Input: part model. Units: mm. Frame: model coordinates. Give positions to 0.01 mm unless a question says otherwise; leave off trailing zeros. Loops run counter-clockwise (first coordinate to the right, second up) from the corner with the lowest first, then second, coordinate; pieces in that order, holes last. Notation, with made-up numbers: (-13, 56.5) -> (4, 56.5) arc R14 cw to (4, 83.5) -> close; hole circle Ø2 at (-4, 89.25). An arc over 180 degrees is marked (long way). Answer in a Markdown table with one row per item. Add a question column.
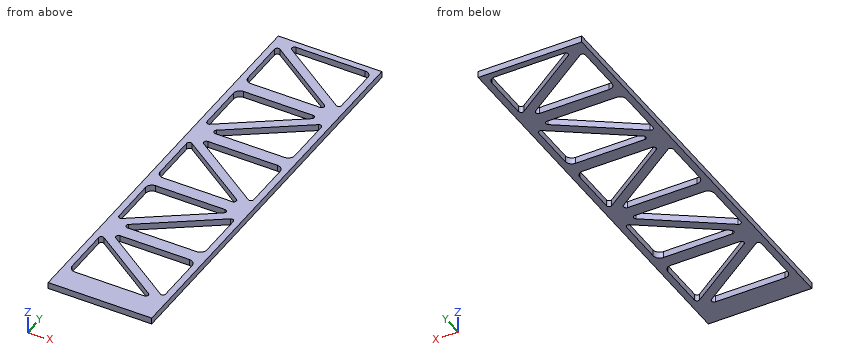
```python
from build123d import *

# Parameters (mm, degrees)
MODEL_W             = 101.6
MODEL_H             = 398.78
BOSS_EXTRUDE1_DEPTH = 6.35


with BuildPart() as part:
    # Model → Boss-Extrude1 (new body)
    with BuildSketch(Plane.XY):
        with Locations((50.8, 199.39)):
            Rectangle(MODEL_W, MODEL_H)
        with BuildLine():
            Line((88.9, 87.63), (20.83121403, 87.63))
            ThreePointArc((20.83121403, 87.63), (18.406749642, 85.847345646), (19.385420684, 83.001631833))
            Line((19.385420684, 83.001631833), (91.264206654, 33.239395393))
            ThreePointArc((91.264206654, 33.239395393), (93.888830968, 33.077884107), (95.25, 35.32776356))
            Line((95.25, 35.32776356), (95.25, 81.28))
            ThreePointArc((95.25, 81.28), (93.390128061, 85.770128061), (88.9, 87.63))
        make_face(mode=Mode.SUBTRACT)
        with BuildLine():
            Line((6.35, 157.48), (6.35, 111.52776356))
            ThreePointArc((6.35, 111.52776356), (7.711169032, 109.277884107), (10.335793346, 109.439395393))
            Line((10.335793346, 109.439395393), (82.214579316, 159.201631833))
            ThreePointArc((82.214579316, 159.201631833), (83.193250358, 162.047345646), (80.76878597, 163.83))
            Line((80.76878597, 163.83), (12.7, 163.83))
            ThreePointArc((12.7, 163.83), (8.209871939, 161.970128061), (6.35, 157.48))
        make_face(mode=Mode.SUBTRACT)
        with BuildLine():
            Line((88.9, 240.03), (20.83121403, 240.03))
            ThreePointArc((20.83121403, 240.03), (18.406749642, 238.247345646), (19.385420684, 235.401631833))
            Line((19.385420684, 235.401631833), (91.264206654, 185.639395393))
            ThreePointArc((91.264206654, 185.639395393), (93.888830968, 185.477884107), (95.25, 187.72776356))
            Line((95.25, 187.72776356), (95.25, 233.68))
            ThreePointArc((95.25, 233.68), (93.390128061, 238.170128061), (88.9, 240.03))
        make_face(mode=Mode.SUBTRACT)
        with BuildLine():
            Line((12.7, 176.53), (80.76878597, 176.53))
            ThreePointArc((80.76878597, 176.53), (83.193250358, 178.312654354), (82.214579316, 181.158368167))
            Line((82.214579316, 181.158368167), (10.335793346, 230.920604607))
            ThreePointArc((10.335793346, 230.920604607), (7.711169032, 231.082115893), (6.35, 228.83223644))
            Line((6.35, 228.83223644), (6.35, 182.88))
            ThreePointArc((6.35, 182.88), (8.209871939, 178.389871939), (12.7, 176.53))
        make_face(mode=Mode.SUBTRACT)
        with BuildLine():
            Line((91.264206654, 154.720604607), (19.385420684, 104.958368167))
            ThreePointArc((19.385420684, 104.958368167), (18.406749642, 102.112654354), (20.83121403, 100.33))
            Line((20.83121403, 100.33), (88.9, 100.33))
            ThreePointArc((88.9, 100.33), (93.390128061, 102.189871939), (95.25, 106.68))
            Line((95.25, 106.68), (95.25, 152.63223644))
            ThreePointArc((95.25, 152.63223644), (93.888830968, 154.882115893), (91.264206654, 154.720604607))
        make_face(mode=Mode.SUBTRACT)
        with BuildLine():
            Line((6.35, 309.88), (6.35, 263.92776356))
            ThreePointArc((6.35, 263.92776356), (7.711169032, 261.677884107), (10.335793346, 261.839395393))
            Line((10.335793346, 261.839395393), (82.214579316, 311.601631833))
            ThreePointArc((82.214579316, 311.601631833), (83.193250358, 314.447345646), (80.76878597, 316.23))
            Line((80.76878597, 316.23), (12.7, 316.23))
            ThreePointArc((12.7, 316.23), (8.209871939, 314.370128061), (6.35, 309.88))
        make_face(mode=Mode.SUBTRACT)
        with BuildLine():
            Line((88.9, 392.43), (20.83121403, 392.43))
            ThreePointArc((20.83121403, 392.43), (18.406749642, 390.647345646), (19.385420684, 387.801631833))
            Line((19.385420684, 387.801631833), (91.264206654, 338.039395393))
            ThreePointArc((91.264206654, 338.039395393), (93.888830968, 337.877884107), (95.25, 340.12776356))
            Line((95.25, 340.12776356), (95.25, 386.08))
            ThreePointArc((95.25, 386.08), (93.390128061, 390.570128061), (88.9, 392.43))
        make_face(mode=Mode.SUBTRACT)
        with BuildLine():
            Line((12.7, 328.93), (80.76878597, 328.93))
            ThreePointArc((80.76878597, 328.93), (83.193250358, 330.712654354), (82.214579316, 333.558368167))
            Line((82.214579316, 333.558368167), (10.335793346, 383.320604607))
            ThreePointArc((10.335793346, 383.320604607), (7.711169032, 383.482115893), (6.35, 381.23223644))
            Line((6.35, 381.23223644), (6.35, 335.28))
            ThreePointArc((6.35, 335.28), (8.209871939, 330.789871939), (12.7, 328.93))
        make_face(mode=Mode.SUBTRACT)
        with BuildLine():
            Line((12.7, 24.13), (80.76878597, 24.13))
            ThreePointArc((80.76878597, 24.13), (83.193250358, 25.912654354), (82.214579316, 28.758368167))
            Line((82.214579316, 28.758368167), (10.335793346, 78.520604607))
            ThreePointArc((10.335793346, 78.520604607), (7.711169032, 78.682115893), (6.35, 76.43223644))
            Line((6.35, 76.43223644), (6.35, 30.48))
            ThreePointArc((6.35, 30.48), (8.209871939, 25.989871939), (12.7, 24.13))
        make_face(mode=Mode.SUBTRACT)
        with BuildLine():
            Line((91.264206654, 307.120604607), (19.385420684, 257.358368167))
            ThreePointArc((19.385420684, 257.358368167), (18.406749642, 254.512654354), (20.83121403, 252.73))
            Line((20.83121403, 252.73), (88.9, 252.73))
            ThreePointArc((88.9, 252.73), (93.390128061, 254.589871939), (95.25, 259.08))
            Line((95.25, 259.08), (95.25, 305.03223644))
            ThreePointArc((95.25, 305.03223644), (93.888830968, 307.282115893), (91.264206654, 307.120604607))
        make_face(mode=Mode.SUBTRACT)
    extrude(amount=BOSS_EXTRUDE1_DEPTH)


solid = part.part
```
1) Section B-B on z = 2.5. State how many separate pieces and enclosed holes the cut face has, and give its area (3 significant figures).
2) Material intervals for line 1 along X through (y, z) = (196, 3.25); line 2 along X through (y, z) = (52, 2); line 3 along Y through (x, z) = (15, 0.5), sorted ascending.
3) Section A-A on y = 59.5. Output: boundary loops of the cut face in (x, z).
Working result:
| question | item | result |
|---|---|---|
| 1 | separate pieces | 1 |
| 1 | enclosed holes | 10 |
| 1 | area | 17,200 mm2 |
| 2 | line 1 | x = 0 to 6.35, 60.78 to 76.3, 95.25 to 101.6 |
| 2 | line 2 | x = 0 to 6.35, 48.64 to 64.17, 95.25 to 101.6 |
| 2 | line 3 | y = 0 to 24.13, 75.29 to 112.67, 163.83 to 176.53, 227.69 to 265.07, 316.23 to 328.93, 380.09 to 398.78 |
| 3 | outline | (0, 0) -> (6.35, 0) -> (6.35, 6.35) -> (0, 6.35) -> close; (37.81, 0) -> (53.33, 0) -> (53.33, 6.35) -> (37.81, 6.35) -> close; (95.25, 0) -> (101.6, 0) -> (101.6, 6.35) -> (95.25, 6.35) -> close |
